Could you check a few things on this model? Use its own coordinates, in mm. A direction names the side the tool comes from. Round coordinates to 2 decimals unless told otherwise and drop trailing zeros. Order: outer loops, then holes, each group sorted by start corner. A loop starts at its lowest first (then second) coordinate and runs counter-clockwise, first axis right, second up. Notation, with made-up numbers: M -38.75,10 L 9.25,10 A20 ccw 9.25,30 Z; hole C 81,41.5 d1. An arc over 180 degrees is marked long. Write each question's results on one line, items separated by ' | '. Start each with the question number.
1. Suppose I cut it at D-D on x = 4. Write out the boundary of the cut face in (y, z).
2. Suppose I cut it at A-A on x = -25. Write out the boundary of the cut face in (y, z).
3. Suppose I cut it at C-C on y = 1.6. Write out the boundary of the cut face in (x, z).
4. We'd pull the mould along Z, two halves only. Please class faces 3 (the flat face through (-19, 1, -26.5)), 4 (the flat face through (-29, 1, 0)), 5 (the cylindrical face through (-23.4, 1, -21.3)): released by +Z, released by -Z, zero draft, split by the parting line, or undercut.
5. Please list where these lines run through material, in increasing order: L1, parallel to Z at x = 25, y = 1.95; L2, parallel to X at y = 0.5, z = 22.5; L3, parallel to Z at x = -25.5, y = 1.2.
6. For faces 1 (the flat face through (9, 1, -24)), 2 (the cylindrical face through (26.474, 0.986, 21.148)), which set-ups out of +Z, -Z, +X, -X, +Y, -Y let a thin tool reach every point of the face, with its end or its side?
7. Suppose I cut it at B-B on z = 22.5. Write out the boundary of the cut face in (x, y), and give its area (3 significant figures).
from build123d import *

# Parameters (mm, degrees)
SKETCH1_W                 = 58
SKETCH1_H                 = 53
BOSS_EXTRUDE1_DEPTH       = 2
F_4_0MM_DOWEL_HOLE1_D     = 4
F_4_0MM_DOWEL_HOLE1_DEPTH = 2
SKETCH4_W                 = 18
SKETCH4_H                 = 5
CUT_EXTRUDE1_DEPTH        = 2


with BuildPart() as part:
    # Sketch1 → Boss-Extrude1 (new body)
    with BuildSketch(Plane(origin=(0, 0, 0), x_dir=(1, 0, 0), z_dir=(0, 1, 0))):
        Rectangle(SKETCH1_W, SKETCH1_H)
    extrude(amount=BOSS_EXTRUDE1_DEPTH)

    # Ø4.0mm Dowel Hole1
    with Locations(Plane(origin=(0, 2, 0), x_dir=(1, 0, 0), z_dir=(0, 1, 0))):
        with Locations((25, 22.5), (-25, 22.5), (-25, -22.5), (25, -22.5)):
            Hole(F_4_0MM_DOWEL_HOLE1_D / 2, depth=F_4_0MM_DOWEL_HOLE1_DEPTH)

    # Sketch4 → Cut-Extrude1 (cut)
    with BuildSketch(Plane(origin=(0, 2, 0), x_dir=(1, 0, 0), z_dir=(0, 1, 0))):
        with Locations((0, 24)):
            Rectangle(SKETCH4_W, SKETCH4_H)
    extrude(amount=-CUT_EXTRUDE1_DEPTH, mode=Mode.SUBTRACT)


solid = part.part
Filled sheet:
1) outline: M 0,-21.5 L 2,-21.5 L 2,26.5 L 0,26.5 Z
2) outline: M 0,-26.5 L 2,-26.5 L 2,-24.5 L 0,-24.5 Z; M 0,-20.5 L 2,-20.5 L 2,20.5 L 0,20.5 Z; M 0,24.5 L 2,24.5 L 2,26.5 L 0,26.5 Z
3) outline: M -29,-26.5 L -9,-26.5 L -9,-21.5 L 9,-21.5 L 9,-26.5 L 29,-26.5 L 29,26.5 L -29,26.5 Z; hole C -25,-22.5 d4; hole C -25,22.5 d4; hole C 25,-22.5 d4; hole C 25,22.5 d4
4) face 3: released by -Z | face 4: zero draft | face 5: undercut
5) L1: z = -26.5 to -24.5, -20.5 to 20.5, 24.5 to 26.5 | L2: x = -29 to -27, -23 to 23, 27 to 29 | L3: z = -26.5 to -24.44, -20.56 to 20.56, 24.44 to 26.5
6) face 1: -Z, +Y, -Y | face 2: +Y, -Y
7) outline: M -29,0 L -27,0 L -27,2 L -29,2 Z; M -23,0 L 23,0 L 23,2 L -23,2 Z; M 27,0 L 29,0 L 29,2 L 27,2 Z | area: 100 mm^2
